```python
from build123d import *

# Parameters (mm, degrees)
SKETCH_1_R      = 1.65
EXTRUDE_1_DEPTH = 3
EXTRUDE_2_DEPTH = 3


with BuildPart() as part:
    # 草图1 → 凸台-拉伸1 (new body)
    with BuildSketch(Plane.XY):
        with BuildLine():
            Line((0, 0), (20, 0))
            Line((20, 0), (20, 33))
            ThreePointArc((20, 33), (10, 43), (0, 33))
            Line((0, 33), (0, 0))
        make_face()
        with Locations((10, 33)):
            Circle(SKETCH_1_R, mode=Mode.SUBTRACT)
    extrude(amount=EXTRUDE_1_DEPTH)

    # 草图5 → 凸台-拉伸2 (add)
    with BuildSketch(Plane(origin=(0, 0, 0), x_dir=(-1, 0, 0), z_dir=(0, 0, -1))):
        Polygon((0, 33), (0, 20), (18, 20), (16.748242373, 33), align=None)
    extrude(amount=-EXTRUDE_2_DEPTH)


solid = part.part
```
Read the model definition and answer for the solid it produces. Units are mm, in the model's axes. A direction names the side the tool comes from. Coordinates: 2 decimals unless noted, no trailing zeros. Loops run counter-clockwise (first coordinate to the right, second up) from the corner with the lowest first, then second, coordinate; pieces in that order, holes last. Notation, with made-up numbers: (68, 27.25) -> (100, 27.25) arc R27 cw to (100, 46.25) -> close; hole circle Ø11 at (72.25, 28.25). An arc over 180 degrees is marked (long way). Return JSON: item names as keys, results as strings.
Item 1: For a pull along Y with two mould halves and no side action, classify faces 4 (the flat face through (20, 16, 1)), 5 (the cylindrical face through (10.89, 34.39, 1.48)), 6 (the flat face through (10, 0, 1)) as +Y half, -Y half, draft (parallel to the pull), parting line (faces both ways), or undercut.
Answers:
{"face 4": "draft", "face 5": "undercut", "face 6": "-Y half"}
Item 2: Find section D-D (x = -14). Determine the outline of the cut face in (y, z).
Answers:
{"outline": "(20, 0) -> (33, 0) -> (33, 3) -> (20, 3) -> close"}
Item 3: Find section C-C (y = 11.5). Determine the outline of the cut face in (x, z), plus the area to 3 significant figures.
Answers:
{"outline": "(0, 0) -> (20, 0) -> (20, 3) -> (0, 3) -> close", "area": "60.0 mm2"}
Item 4: Find section B-B (z = 2.1). Determine the outline of the cut face in (x, y).
Answers:
{"outline": "(-18, 20) -> (0, 20) -> (0, 0) -> (20, 0) -> (20, 33) arc R10 ccw to (0, 33) -> (-16.75, 33) -> close; hole circle Ø3.3 at (10, 33)"}
Item 5: Find section A-A (x = 10). Determine the outline of the cut face in (y, z).
Answers:
{"outline": "(0, 0) -> (31.35, 0) -> (31.35, 3) -> (0, 3) -> close; (34.65, 0) -> (43, 0) -> (43, 3) -> (34.65, 3) -> close"}
Item 6: Find the intervals of material crossed by probe 1 along Y at (x, z) = (10, 2.1); probe 2 along X at (y, z) = (17.5, 0.2); probe 3 along Y at (x, z) = (-8.5, 2), in increasing order.
Answers:
{"probe 1": "y = 0 to 31.35, 34.65 to 43", "probe 2": "x = 0 to 20", "probe 3": "y = 20 to 33"}
Item 7: For faces 1 (the flat face through (-8, 33, 1)), 2 (the flat face through (5, 22, 3)), 3 (the flat face through (0, 10, 1)), determine the directions among +Z, -Z, +X, -X, +Y, -Y from which every point of the face is accessible in a straight line to the end or side of a thin tool.
Answers:
{"face 1": "+Z, -Z, -X, +Y", "face 2": "+Z, +X, -X, +Y, -Y", "face 3": "+Z, -Z, -X, -Y"}
Item 8: Flat-ended cylindrical pins translate along their axes: P1, Ø1, axis at y = 9.5, z = 0.5, coming from the -X side; P2, Ø1.5, axis at x = -7.5, z = 1, coming from the -Y side. Find the tip coordinate at first contact, or state that the pin passes through.
Answers:
{"P1": "stops at x = 0", "P2": "stops at y = 20"}
